Can you work these out from the model? Positions are in its coordinate system, mm. A direction names the side the tool comes from. Round coordinates to 2 decimals unless told otherwise and drop trailing zeros. Write each loop counter-clockwise with the first axis right and the second up, starting at its lowest first coordinate (ties: lowest second). Pieces come first, ordered by that corner, then holes.
Q1. If we section it at A-A (y = 0): Please give me the cut outline in (x, z) (3 decimals), plus the area to 3 significant figures.
Q2. If we section it at D-D (z = -12): Please give me the cut outline in (x, y) (3 decimals).
Q3. Please list where these lines run through material, in increasing order: line 1 along Y through (x, z) = (0, -0.5) (3 decimals); line 2 along Z through (x, y) = (120, -112.5); line 3 along X through (y, z) = (-160, 14).
Q4. For faces 1 (the cylindrical face through (16.573, -5.219, -0.493)), 2 (the flat face through (36, 146, 17.25)), 3 (the flat face through (-36, 146, -17.25)), which set-ups out of +Z, -Z, +X, -X, +Y, -Y let a thin tool reach every point of the face, with its end or its side?
Q5. If we section it at C-C (z = 9.5): Please give me the cut outline in (x, y) (3 decimals).
Q6. We'd pull the mould along X, two halves only. Please class faces 4 (the conical face through (158.92, -50.05, 17.48)), 5 (the conical face through (-8.849, 39.851, 34.376)), 6 (the flat face through (-16.2, 7.3, 35.25)): +X half, -X half, draft (parallel to the pull), parting line (faces both ways), or undercut.
Q7. I'm going to push flat-ended pins straight in: pin 1 Ø10 at (y, z) = (-76, -19.5) entering from +X; pin 2 Ø12 at (y, z) = (-58, -11.5) entering from +X; pin 3 Ø8 at (y, z) = (-57.5, 3) entering from -X. Where does each tip first touch, or does it pass through?
from build123d import *


with BuildPart() as part:
    # Sketch1 → Revolve1 (revolve)
    with BuildSketch(Plane(origin=(0, 0, 0), x_dir=(0, 0, -1), z_dir=(1, 0, 0)), mode=Mode.PRIVATE) as revolve1_sk:
        with BuildLine():
            Line((35.25, 35.25), (17.25, 150))
            Line((17.25, 150), (17.25, 165))
            Line((17.25, 165), (22, 198.2))
            ThreePointArc((22, 198.2), (0, 203.2), (-22, 198.2))
            Line((-22, 198.2), (-17.25, 165))
            Line((-17.25, 165), (-17.25, 150))
            Line((-17.25, 150), (-35.25, 35.25))
            Line((-35.25, 35.25), (-35.25, 17.375))
            Line((-35.25, 17.375), (35.25, 17.375))
            Line((35.25, 17.375), (35.25, 35.25))
        make_face()
    revolve(revolve1_sk.sketch.rotate(Axis((0, 0, 0), (0, 0, -1)), 90), axis=Axis((0, 0, 0), (0, 0, -1)))


solid = part.part
A:
1. outline: (-198.2, -22) - (-165, -17.25) - (-150, -17.25) - (-35.25, -35.25) - (-17.375, -35.25) - (-17.375, 35.25) - (-35.25, 35.25) - (-150, 17.25) - (-165, 17.25) - (-198.2, 22) arc R50.9 ccw to start; (17.375, -35.25) - (35.25, -35.25) - (150, -17.25) - (165, -17.25) - (198.2, -22) arc R50.9 ccw to (198.2, 22) - (165, 17.25) - (150, 17.25) - (35.25, 35.25) - (17.375, 35.25) - close
1. area: 18,500 mm2
2. outline: circle Ø403.53 at (0, 0); hole circle Ø34.75 at (0, 0)
3. line 1: y = -203.198 to -17.375, 17.375 to 203.198
3. line 2: z = -17.25 to 17.25
3. line 3: x = -122.05 to 122.05
4. face 1: +Z, -Z
4. face 2: +Z
4. face 3: -Z
5. outline: circle Ø404.611 at (0, 0); hole circle Ø34.75 at (0, 0)
6. face 4: undercut
6. face 5: undercut
6. face 6: draft
7. pin 1: stops at x = 187.09
7. pin 2: stops at x = 195.48
7. pin 3: stops at x = -195.96
